Work out the finished part from the listing and answer in its coordinate system (mm). A direction names the side the tool comes from. Give positions to 0.01 mm unless a question says otherwise; leave off trailing zeros. Order: outer loops, then holes, each group sorted by start corner. A loop starts at its lowest first (then second) coordinate and runs counter-clockwise, first axis right, second up. Notation, with made-up numbers: (46.5, 44) - (102.5, 44) arc R22 ccw to (102.5, 63) - close; hole circle Ø2 at (-25.5, -25.5). An arc over 180 degrees is marked (long way). Write each question's results on one line, items separated by ' | '.
from build123d import *

# Parameters (mm, degrees)
SKETCH1_R               = 83.4771
SKETCH1_R_2             = 72.5043
BOSS_EXTRUDE1_DEPTH     = 82.55
SKETCH2_W               = 47.625
SKETCH2_H               = 114.3
CUT_EXTRUDE1_DEPTH      = 84.4771
SKETCH3_W               = 76.2
SKETCH3_H               = 25.4
CUT_EXTRUDE2_DEPTH      = 84.4771
CUT_EXTRUDE2_DEPTH_BACK = 84.4771
SKETCH4_R               = 22.225
CUT_EXTRUDE3_DEPTH      = 97.1771
SKETCH6_W               = 76.2
SKETCH6_H               = 3.175
CUT_EXTRUDE4_DEPTH      = 84.4771001
CUT_EXTRUDE4_DEPTH_BACK = 84.4771001


with BuildPart() as part:
    # Sketch1 → Boss-Extrude1 (new body, symmetric)
    with BuildSketch(Plane.XY):
        Circle(SKETCH1_R)
        Circle(SKETCH1_R_2, mode=Mode.SUBTRACT)
    extrude(amount=BOSS_EXTRUDE1_DEPTH, both=True)

    # Sketch2 → Cut-Extrude1 (cut, through all)
    with BuildSketch(Plane(origin=(0, 0, 0), x_dir=(1, 0, 0), z_dir=(0, 1, 0))):
        with Locations((0, -25.4)):
            Rectangle(SKETCH2_W, SKETCH2_H)
    extrude(amount=CUT_EXTRUDE1_DEPTH, mode=Mode.SUBTRACT)

    # Sketch3 → Cut-Extrude2 (cut, two sides)
    with BuildSketch(Plane(origin=(0, 0, 0), x_dir=(0, 0, -1), z_dir=(1, 0, 0))) as cut_extrude2_sk:
        with Locations((12.7, 0)):
            Rectangle(SKETCH3_W, SKETCH3_H)
    extrude(amount=CUT_EXTRUDE2_DEPTH, mode=Mode.SUBTRACT)
    extrude(cut_extrude2_sk.sketch, amount=-CUT_EXTRUDE2_DEPTH_BACK, mode=Mode.SUBTRACT)

    # Sketch4 → Cut-Extrude3 (cut, through all)
    with BuildSketch(Plane(origin=(0, -12.7, 0), x_dir=(1, 0, 0), z_dir=(0, 1, 0))):
        with Locations((-82.505370882, 12.7)):
            Circle(SKETCH4_R)
        with Locations((82.505370882, 12.7)):
            Circle(SKETCH4_R)
    extrude(amount=CUT_EXTRUDE3_DEPTH, mode=Mode.SUBTRACT)

    # Sketch6 → Cut-Extrude4 (cut, two sides)
    with BuildSketch(Plane(origin=(0, 0, 0), x_dir=(0, 0, -1), z_dir=(1, 0, 0))) as cut_extrude4_sk:
        with Locations((12.7, 14.2875)):
            Rectangle(SKETCH6_W, SKETCH6_H)
    extrude(amount=CUT_EXTRUDE4_DEPTH, mode=Mode.SUBTRACT)
    extrude(cut_extrude4_sk.sketch, amount=-CUT_EXTRUDE4_DEPTH_BACK, mode=Mode.SUBTRACT)


solid = part.part
1. Given P1, Ø2, axis at x = -15, z = 6.5, coming from the +Y side; P2, Ø6, axis at x = -33, z = -37.5, coming from the +Y side; P3, Ø5.5, axis at x = 74.5, z = 15.5, coming from the -Y side, each flat-ended and moving along its own axis, determine where each tip first touches the part or whether it passes through.
Answer list:
P1: y = -70.72 | P2: y = 77.9 | P3: y = -42.67
2. A cutting plane is placed at A-A, the plane z = 18. Write down the section's boundary in (x, y) (1 decimal).
Answer list:
outline: (-82.5, -12.7) arc R83.5 ccw to (82.5, -12.7) - (71.4, -12.7) arc R72.5 cw to (-71.4, -12.7) - close; (-82, 15.9) - (-70.7, 15.9) arc R72.5 cw to (-23.8, 68.5) - (-23.8, 80) arc R83.5 ccw to start; (23.8, 68.5) arc R72.5 cw to (70.7, 15.9) - (82, 15.9) arc R83.5 ccw to (23.8, 80) - close
3. Determine the mould class of faces 1 (the face through (33.5, -64.3, -1.2)), 2 (the face through (77, 1, 25.4)), 3 (the face through (23.812, 74, 26)), 4 (the face through (-60.286, 41.174, -12.219)) for opening direction X: +X half, -X half, draft (parallel to the pull), parting line (faces both ways), or undercut.
Answer list:
face 1: undercut | face 2: draft | face 3: undercut | face 4: -X half
4. A cutting plane is placed at B-B, the plane x = 0. Write down the section's boundary in (y, z), then the cut area to 3 significant figures.
Answer list:
outline: (-83.48, -82.55) - (-72.5, -82.55) - (-72.5, 82.55) - (-83.48, 82.55) - close; (72.5, -82.55) - (83.48, -82.55) - (83.48, -31.75) - (72.5, -31.75) - close | area: 2,370 mm^2
5. A cutting plane is placed at D-D, the plane z = -41. Write down the section's boundary in (x, y) (3 decimals).
Answer list:
outline: (-82.505, -12.7) arc R83.477 ccw to (82.505, -12.7) - (71.383, -12.7) arc R72.504 cw to (-71.383, -12.7) - close; (-81.954, 15.875) - (-70.745, 15.875) arc R72.504 cw to (70.745, 15.875) - (81.954, 15.875) arc R83.477 ccw to start
6. A tool of negligible diameter and unlimited length cuts with its end or side. For faces 5 (the face through (-25.1, 68.4, -82.55)), 6 (the face through (60.286, 41.17, -13.181)), 7 (the face through (77, 1, -50.8)), 8 (the face through (0, 76, -31.75)), 9 (the face through (38.52, -74.06, 1.16)), from which of +Z, -Z, +X, -X, +Y, -Y can it reach the whole face along a straight path? Write none if from no direction.
Answer list:
face 5: -Z, +X, -X, +Y, -Y | face 6: +X, +Y | face 7: +X, -X | face 8: +Z, +Y | face 9: +Z, -Z
7. Straight lines are drawn through the part: line 1 (Y direction, x = 0, z = -35); line 2 (Y direction, x = 0, z = -21). For each, find the intervals that lie inside material, in ascending order. Write a range as [from, to].
Answer list:
line 1: [-83.48, -72.5], [72.5, 83.48] | line 2: [-83.48, -72.5]
8. A cutting plane is placed at C-C, the plane y = 40. Write down the section's boundary in (x, z) (3 decimals), then the cut area to 3 significant figures.
Answer list:
outline: (-73.27, -82.55) - (-60.472, -82.55) - (-60.472, -15.613) arc R22.225 cw to (-73.27, -32.915) - close; (-73.27, 7.515) arc R22.225 cw to (-60.472, -9.787) - (-60.472, 82.55) - (-73.27, 82.55) - close; (60.472, -82.55) - (73.27, -82.55) - (73.27, -32.915) arc R22.225 cw to (60.472, -15.613) - close; (60.472, -9.787) arc R22.225 cw to (73.27, 7.515) - (73.27, 82.55) - (60.472, 82.55) - close | area: 3,470 mm^2
